from build123d import *

# Parameters (mm, degrees)
SKETCH_1_R          = 12.625
SKETCH_1_R_2        = 7.625
EXTRUDE_1_DEPTH     = 22.5
EXTRUDE_2_DEPTH     = 17.499994584
CUT_EXTRUDE_1_DEPTH = 70.296381035
FILLET_1_R          = 3
SKETCH_4_R          = 1.6
CUT_EXTRUDE_5_DEPTH = 66.731667206
SKETCH_5_R          = 2.75
CUT_EXTRUDE_6_DEPTH = 3


with BuildPart() as part:
    # 草图1 → 凸台-拉伸1 (new body)
    with BuildSketch(Plane.XY):
        Circle(SKETCH_1_R)
        Circle(SKETCH_1_R_2, mode=Mode.SUBTRACT)
    extrude(amount=-EXTRUDE_1_DEPTH)

    # 草图2 → 凸台-拉伸2 (add)
    with BuildSketch(Plane.XY):
        with BuildLine():
            Line((11.206194864, -5.814793347), (-14.125578135, -54.633860081))
            Line((-14.125578135, -54.633860081), (-36.537967862, -43.004273386))
            Line((-36.537967862, -43.004273386), (-11.206194864, 5.814793347))
            ThreePointArc((-11.206194864, 5.814793347), (-5.814793347, -11.206194864), (11.206194864, -5.814793347))
        make_face()
    extrude(amount=-EXTRUDE_2_DEPTH)

    # 草图3 → 切除-拉伸1 (cut, through all)
    with BuildSketch(Plane(origin=(-11.206194864, 5.814793347, 0), x_dir=(0, 0, 1), z_dir=(-0.8876193951581107, 0.46057769088303635, 0))):
        Polygon((-8.749997893, -55), (-8.749997893, -42.655440917), (0, -27.5), (0, -55), align=None)
    extrude(amount=-CUT_EXTRUDE_1_DEPTH, mode=Mode.SUBTRACT)

    # 圆角1
    fillet_1_edges = [part.edges().sort_by_distance(p)[0] for p in [
        (-14.125578135, -54.633860081, -13.124996239),
        (-36.537967862, -43.004273386, -13.124996239),
    ]]
    fillet(fillet_1_edges, radius=FILLET_1_R)

    # 草图4 → 切除-拉伸5 (cut, through all)
    with BuildSketch(Plane.XY.offset(-8.749997893)):
        with Locations((-13.957898202, -43.454777675)):
            Circle(SKETCH_4_R)
        with Locations((-27.494093978, -36.430967889)):
            Circle(SKETCH_4_R)
    extrude(amount=-CUT_EXTRUDE_5_DEPTH, mode=Mode.SUBTRACT)

    # 草图5 → 切除-拉伸6 (cut)
    with BuildSketch(Plane.XY.offset(-8.749997893)):
        with Locations((-13.957898202, -43.454777675)):
            Circle(SKETCH_5_R)
        with Locations((-27.494093978, -36.430967889)):
            Circle(SKETCH_5_R)
    extrude(amount=-CUT_EXTRUDE_6_DEPTH, mode=Mode.SUBTRACT)


solid = part.part
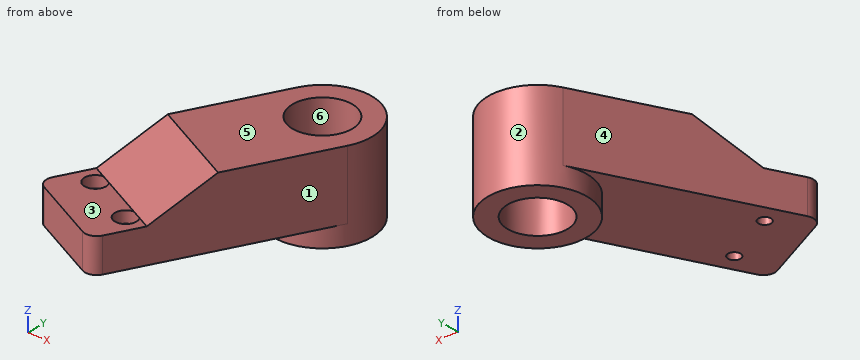
Source: CAD feature listing. Evaluate the final solid. Frame: model axes, mm. Face numbers are marked on the shaded views. A direction names the side the tool comes from. Round coordinates to 2 decimals unless told otherwise and drop trailing zeros. Loops run counter-clockwise (first coordinate to the right, second up) from the corner with the lowest first, then second, coordinate; pieces in that order, holes last. Notation, with made-up numbers: M 57.25,64.25 L 115.25,64.25 A33 cw 115.25,103.25 Z; hole C 26,48 d4. An arc over 180 degrees is marked long. Return JSON: item names as keys, results as strings. Group by question number.
1. Reachability of the marked faces 1, 2 and 3 from +Z, -Z, +X, -X, +Y, -Y: full face, straight path, thin tool, end or side. Return the list, or none.
2. Section query C-C on z = -15. Output: boundary loops of the cut face in (x, y) (3 decimals), and give its area (3 significant figures).
3. Mould query, pull axis X, two halves, no side actions, for the marked faces 4, 5 and 6. Classes: released by +X, released by -X, zero draft, split by the parting line, or undercut.
4. Section query B-B on x = 0. Output: boundary loops of the cut face in (y, z) (3 decimals), and give its area (3 significant figures).
5. Section query A-A on y = 0. Output: boundary loops of the cut face in (x, z) (3 decimals), and give its area (3 significant figures).
6. Material intervals for line 1 along Z through (x, y) = (-14, -45.5); line 2 along Y through (x, z) = (5, -3.25); line 3 along Z through (x, y) = (-2, -13.5), sorted ascending. Write a range as from..to.
7. Section query D-D on z = -7.75. Output: boundary loops of the cut face in (x, y) (3 decimals).
8. Pin query (flat end, axial travel): pin 1 (4 mm diameter, centred on x = -11.5, y = -11, fed in from -Z); pin 2 (3 mm diameter, centred on x = 5.5, z = -9.5, fed in from +Y); pin 3 (3.5 mm diameter, centred on x = -13.96, y = -43.45, fed in from +Z). Return the tip coordinate at first contact, or that it passes through.
Checks:
{
 "1": {"face 1": "+Z, -Z, +X, -Y", "face 2": "-Z", "face 3": "+Z, -X, -Y"},
 "2": {"outline": "M -35.156,-40.341 A3 ccw -33.875,-44.386 L -16.788,-53.252 A3 ccw -12.744,-51.971 L 11.206,-5.815 A12.625 ccw -11.206,5.815 Z; hole C -27.494,-36.431 d3.2; hole C -13.958,-43.455 d3.2; hole C 0,0 d15.25", "area": "1,440 mm²"},
 "3": {"face 4": "released by -X", "face 5": "zero draft", "face 6": "undercut"},
 "4": {"outline": "M -27.411,-17.5 L -12.625,-17.5 L -12.625,-22.5 L -7.625,-22.5 L -7.625,0 L -27.411,0 Z; M 7.625,-22.5 L 12.625,-22.5 L 12.625,0 L 7.625,0 Z", "area": "484 mm²"},
 "5": {"outline": "M -14.223,-17.5 L -12.625,-17.5 L -12.625,-22.5 L -7.625,-22.5 L -7.625,0 L -14.223,0 Z; M 7.625,-22.5 L 12.625,-22.5 L 12.625,0 L 7.625,0 Z", "area": "253 mm²"},
 "6": {"line 1": "z = -17.5..-11.75", "line 2": "y = -17.78..-5.76, 5.76..11.59", "line 3": "z = -17.5..0"},
 "7": {"outline": "M -30.055,-30.51 L -7.642,-42.139 L 11.206,-5.815 A12.625 ccw -11.206,5.815 Z; hole C 0,0 d15.25"},
 "8": {"pin 1": "stops at z = -17.5", "pin 2": "stops at y = 11.97", "pin 3": "stops at z = -11.75"}
}
